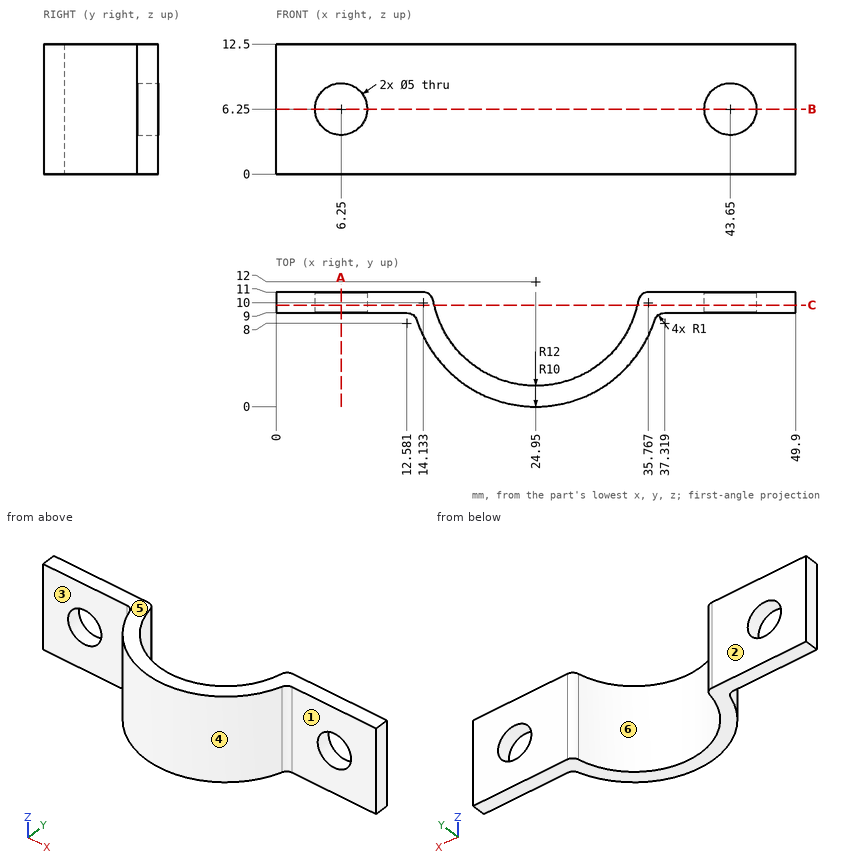
Here's the drawing with two shaded views (mm, measured from the low corner). I have some questions. A direction names the side the tool comes from. Round coordinates to 2 decimals unless told otherwise and drop trailing zeros. Write each loop counter-clockwise with the first axis right and the second up, starting at its lowest first coordinate (ties: lowest second). Pieces come first, ordered by that corner, then holes.
(1) Suppose I cut it at C-C on y = 9.75. Write out the boundary of the cut face in (x, z), and give its area (3 significant figures).
Findings below:
outline: (0, 0) - (15.21, 0) - (15.21, 12.5) - (0, 12.5) - close; (34.69, 0) - (49.9, 0) - (49.9, 12.5) - (34.69, 12.5) - close; hole circle Ø5 at (6.25, 6.25); hole circle Ø5 at (43.65, 6.25)
area: 341 mm2
(2) Which directions (+Z, -Z, +X, -X, +Y, -Y) give clear straight access to the entire face, cutting with the end or side of a thin tool? Please do the marked faces 1, 2 and 3.
Findings below:
face 1: +Z, -Z, +X, -Y
face 2: +Z, -Z, +X, -X, +Y
face 3: +Z, -Z, -X, -Y
(3) Suppose I cut it at A-A on x = 6.25. Write out the boundary of the cut face in (y, z), and give its area (3 significant figures).
Findings below:
outline: (9, 0) - (11, 0) - (11, 3.75) - (9, 3.75) - close; (9, 8.75) - (11, 8.75) - (11, 12.5) - (9, 12.5) - close
area: 15.0 mm2
(4) Suppose I cut it at B-B on z = 6.25. Write out the boundary of the cut face in (x, y).
Findings below:
outline: (0, 9) - (3.75, 9) - (3.75, 11) - (0, 11) - close; (8.75, 9) - (12.58, 9) arc R1 cw to (13.53, 8.31) arc R12 ccw to (36.37, 8.31) arc R1 cw to (37.32, 9) - (41.15, 9) - (41.15, 11) - (35.77, 11) arc R1 ccw to (34.78, 10.18) arc R10 cw to (15.12, 10.18) arc R1 ccw to (14.13, 11) - (8.75, 11) - close; (46.15, 9) - (49.9, 9) - (49.9, 11) - (46.15, 11) - close
(5) If I drill on probe 1 along Z at (x, y) = (6.25, 9.5); probe 2 along X at (y, z) = (10.15, 6.25); probe 3 along Y at (x, z) = (40, 2.25), over which ranges is the centre line in solid material (lowest first)?
Findings below:
probe 1: z = 0 to 3.75, 8.75 to 12.5
probe 2: x = 0 to 3.75, 8.75 to 15.12, 34.78 to 41.15, 46.15 to 49.9
probe 3: y = 9 to 11
(6) Thinking about a two-plate mould opening in X: for the marked faces 4, 5 and 6, which applies, +X half, -X half, draft (parallel to the pull), parting line (faces both ways), or undercut?
Findings below:
face 4: parting line
face 5: draft
face 6: undercut
(7) For pin 1 (4 mm diameter, centred on x = 43.65, z = 6.25, fed in from -Y); pin 2 (6 mm diameter, centred on y = 3.5, z = 8.5, fed in from -X) (1 decimal); pin 3 (6 mm diameter, centred on y = 3, z = 9, fed in from -X); pin 4 (4 mm diameter, centred on x = 43, z = 9, fed in from -Y), each with a flat end and sliding along its axis, tell me the tip position at first contact or that it passes through.
Findings below:
pin 1: passes through
pin 2: stops at x = 14.3
pin 3: stops at x = 14.56
pin 4: stops at y = 9
